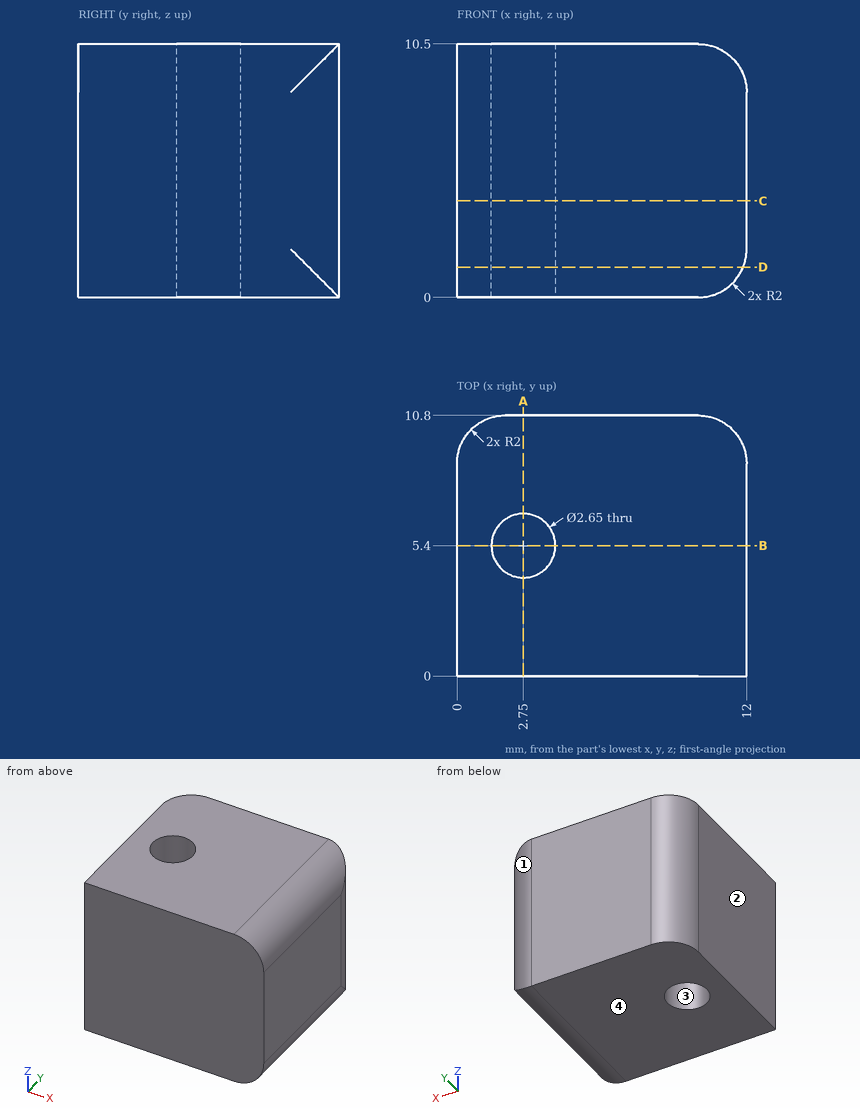
For this review, use the dimensioned drawing (mm, ordinates from the lowest corner) and the shaded views. Round coordinates to 2 decimals unless told otherwise and drop trailing zeros. Order: outer loops, then holes, each group sorted by start corner. A loop starts at its lowest first (then second) coordinate and runs counter-clockwise, first axis right, second up.
1) Consider section D-D (z = 1.25). State the section outline as (x, y) points (3 decimals).
The answers:
outline: (0, 0) - (11.854, 0) - (11.854, 9.55) arc R2 ccw to (10, 10.8) - (2, 10.8) arc R2 ccw to (0, 8.8) - close; hole circle Ø2.65 at (2.75, 5.4)
2) Consider section B-B (y = 5.4). State the section outline as (x, z) points (3 decimals), plus the area to 3 significant figures.
The answers:
outline: (0, 0) - (1.425, 0) - (1.425, 10.5) - (0, 10.5) - close; (4.075, 0) - (10, 0) arc R2 ccw to (12, 2) - (12, 8.5) arc R2 ccw to (10, 10.5) - (4.075, 10.5) - close
area: 96.5 mm2
3) Consider section A-A (x = 2.75). State the section outline as (y, z) points (3 decimals).
The answers:
outline: (0, 0) - (4.075, 0) - (4.075, 10.5) - (0, 10.5) - close; (6.725, 0) - (10.8, 0) - (10.8, 10.5) - (6.725, 10.5) - close
4) Consider section C-C (z = 4). State the section outline as (x, y) points (3 decimals), plus the area to 3 significant figures.
The answers:
outline: (0, 0) - (12, 0) - (12, 8.8) arc R2 ccw to (10, 10.8) - (2, 10.8) arc R2 ccw to (0, 8.8) - close; hole circle Ø2.65 at (2.75, 5.4)
area: 122 mm2
5) For L1, parallel to Y at x = 2.75, z = 8 (3 decimals); L2, parallel to X at y = 6, z = 4.75; L3, parallel to X at y = 9, z = 8.75, list the stretches that pass through material, from the lowest coordinate up.
The answers:
L1: y = 0 to 4.075, 6.725 to 10.8
L2: x = 0 to 1.57, 3.93 to 12
L3: x = 0.01 to 11.98
6) Draft analysis for pull direction X (two halves, no side actions). For the marked faces 1, 2, 3 and 4, state which applies: released by +X, released by -X, zero draft, split by the parting line, or undercut.
The answers:
face 1: released by +X
face 2: released by -X
face 3: undercut
face 4: zero draft
7) Clearance check with a flat-ended pin moving along its axis: pin 1 Ø1.6 at (x, y) = (2.75, 5.4) entering from +Z. State where the tip first meets the part, or that it passes through.
The answers:
pin 1: passes through
